```python
from build123d import *

# Parameters (mm, degrees)
SKETCH_1_R          = 9.5
EXTRUDE_1_DEPTH     = 8
SKETCH_1_2_R        = 9.5
EXTRUDE_2_DEPTH     = 8
SKETCH_2_R          = 12
CUT_EXTRUDE_1_DEPTH = 6
SKETCH_3_W          = 20.5
SKETCH_3_H          = 27
CUT_EXTRUDE_2_DEPTH = 4
SKETCH_4_R          = 1.25
CUT_EXTRUDE_3_DEPTH = 5
SKETCH_5_R          = 1.25
CUT_EXTRUDE_4_DEPTH = 7
SKETCH_6_R          = 1.25
CUT_EXTRUDE_5_DEPTH = 7


with BuildPart() as part:
    # Sketch 1 → Extrude 1 (new body)
    with BuildSketch(Plane(origin=(0, 0, 0), x_dir=(1, 0, 0), z_dir=(0, 1, 0))):
        Polygon((-20.5, -13.5), (-20.5, -7.5), (-16.5, -3.5), (-16.5, 3.5), (-20.5, 7.5), (-20.5, 13.5), (41, 13.5), (41, -13.5), align=None)
        with Locations(Location((0, 0, 0), (0, 0, 270))):  # turned: the seam where the file's is
            Circle(SKETCH_1_R, mode=Mode.SUBTRACT)
    extrude(amount=EXTRUDE_1_DEPTH)

    # Sketch 1_2 → Extrude 2 (add)
    with BuildSketch(Plane(origin=(0, 0, 0), x_dir=(1, 0, 0), z_dir=(0, 1, 0))):
        Polygon((-20.5, -13.5), (-20.5, -7.5), (-16.5, -3.5), (-16.5, 3.5), (-20.5, 7.5), (-20.5, 13.5), (41, 13.5), (41, -13.5), align=None)
        with Locations(Location((0, 0, 0), (0, 0, 270))):  # turned: the seam where the file's is
            Circle(SKETCH_1_2_R, mode=Mode.SUBTRACT)
    extrude(amount=EXTRUDE_2_DEPTH)

    # Sketch 2 → Cut-Extrude 1 (cut)
    with BuildSketch(Plane(origin=(0, 8, 0), x_dir=(1, 0, 0), z_dir=(0, 1, 0))):
        with Locations(Location((0, 0, 0), (0, 0, 270))):  # turned: the seam where the file's is
            Circle(SKETCH_2_R)
    extrude(amount=-CUT_EXTRUDE_1_DEPTH, mode=Mode.SUBTRACT)

    # Sketch 3 → Cut-Extrude 2 (cut)
    with BuildSketch(Plane.XZ):
        with Locations((30.75, 0)):
            Rectangle(SKETCH_3_W, SKETCH_3_H)
    extrude(amount=-CUT_EXTRUDE_2_DEPTH, mode=Mode.SUBTRACT)

    # Sketch 4 → Cut-Extrude 3 (cut, through all)
    with BuildSketch(Plane.XZ.offset(-4)):
        with Locations(Location((37, 7.5, 0), (0, 0, 270))):  # turned: the seam where the file's is
            Circle(SKETCH_4_R)
        with Locations(Location((37, -7.5, 0), (0, 0, 90))):  # turned: the seam where the file's is
            Circle(SKETCH_4_R)
    extrude(amount=-CUT_EXTRUDE_3_DEPTH, mode=Mode.SUBTRACT)

    # Sketch 5 → Cut-Extrude 4 (cut)
    with BuildSketch(Plane.XY.offset(13.5)):
        with Locations((-16.5, 3.500018951)):
            Circle(SKETCH_5_R)
        with Locations(Location((16.5, 3.500018951, 0), (0, 0, 180))):  # turned: the seam where the file's is
            Circle(SKETCH_5_R)
    extrude(amount=-CUT_EXTRUDE_4_DEPTH, mode=Mode.SUBTRACT)

    # Sketch 6 → Cut-Extrude 5 (cut)
    with BuildSketch(Plane(origin=(0, 0, -13.5), x_dir=(-1, 0, 0), z_dir=(0, 0, -1))):
        with Locations((16.5, 4)):
            Circle(SKETCH_6_R)
        with Locations(Location((-16.5, 4, 0), (0, 0, 180))):  # turned: the seam where the file's is
            Circle(SKETCH_6_R)
    extrude(amount=-CUT_EXTRUDE_5_DEPTH, mode=Mode.SUBTRACT)


solid = part.part
```
The listing builds one solid part. Answer for the finished solid, in the listing's coordinates (mm). A direction names the side the tool comes from. Give positions to 0.01 mm unless a question says otherwise; leave off trailing zeros. Order: outer loops, then holes, each group sorted by start corner. A loop starts at its lowest first (then second) coordinate and runs counter-clockwise, first axis right, second up. Notation, with made-up numbers: (75.5, 88) - (86.5, 88) arc R18 ccw to (86.5, 97) - close; hole circle Ø11 at (-6, 56). An arc over 180 degrees is marked (long way). Answer in a Markdown table with one row per item. Add a question column.
Q1. Given P1, Ø10, axis at x = 5.5, z = 3.5, coming from the +Y side; P2, Ø1.2, axis at y = 2.5, z = 3.5, coming from the +X side; P3, Ø3, axis at x = -16.5, y = 3.5, coming from the -Z side; P4, Ø3, axis at x = 37, z = 7.5, coming from the -Y side, each flat-ended and moving along its own axis, determine where each tip first touches the part or whether it passes through.
Q2. Find the intervals of material crossed by line 1 along X through (y, z) = (0.7, 0); line 2 along X through (y, z) = (5.3, -7.5); line 3 along X through (y, z) = (6.4, 0), in increasing order. Write a range as [from, to].
Q3. The part is cut by section C-C (z = 0). Determine the outline of the cut face in (x, y), then the cut area to 3 significant figures.
Q4. For a pull along Y with two mould halves and no side action, classify faces 5 (the flat face through (17, 3, 6.5)), 6 (the flat face through (-20.5, 4, -10)), 7 (the flat face through (18, 8, 0)) as released by +Y, released by -Y, zero draft, split by the parting line, or undercut.
Q5. Which of the six approach directions +Z, -Z, +X, -X, +Y, -Y give full straight-line access (tool end or side, diameter ignored) to faces 1 (the cylindrical face through (16.23, 5.22, -10.05)), 2 (the flat face through (31, 4, 0)), 3 (the flat face through (-19, 4, 6)), 4 (the cylindrical face through (-16.77, 2.28, 10.05))?
Q6. The part is cut by section B-B (y = 7.25). Determine the outline of the cut face in (x, z).
Q7. The part is cut by section A-A (x = 37). Determine the outline of the cut face in (y, z).
Q8. The part is cut by section D-D (x = 16.5). Determine the outline of the cut face in (y, z), then the cut area to 3 significant figures.
Determined:
| question | item | result |
|---|---|---|
| 1 | P1 | stops at y = 2 |
| 1 | P2 | stops at x = 20.5 |
| 1 | P3 | stops at z = -13.5 |
| 1 | P4 | stops at y = 4 |
| 2 | line 1 | x = [-16.5, -9.5], [9.5, 20.5] |
| 2 | line 2 | x = [-20.5, -9.37], [9.37, 35.75], [38.25, 41] |
| 2 | line 3 | x = [-16.5, -12], [12, 41] |
| 3 | outline | (-16.5, 0) - (-9.5, 0) - (-9.5, 2) - (-12, 2) - (-12, 8) - (-16.5, 8) - close; (9.5, 0) - (20.5, 0) - (20.5, 4) - (41, 4) - (41, 8) - (12, 8) - (12, 2) - (9.5, 2) - close |
| 3 | area | 196 mm² |
| 4 | face 5 | undercut |
| 4 | face 6 | zero draft |
| 4 | face 7 | released by +Y |
| 5 | face 1 | -Z |
| 5 | face 2 | +Z, -Z, +X, -Y |
| 5 | face 3 | -X, +Y, -Y |
| 5 | face 4 | +Z |
| 6 | outline | (-20.5, -13.5) - (41, -13.5) - (41, 13.5) - (-20.5, 13.5) - (-20.5, 7.5) - (-16.5, 3.5) - (-16.5, -3.5) - (-20.5, -7.5) - close; hole circle Ø24 at (0, 0); hole circle Ø2.5 at (37, -7.5); hole circle Ø2.5 at (37, 7.5) |
| 7 | outline | (4, -13.5) - (8, -13.5) - (8, -8.75) - (4, -8.75) - close; (4, -6.25) - (8, -6.25) - (8, 6.25) - (4, 6.25) - close; (4, 8.75) - (8, 8.75) - (8, 13.5) - (4, 13.5) - close |
| 8 | outline | (0, -13.5) - (2.75, -13.5) - (2.75, -6.5) - (5.25, -6.5) - (5.25, -13.5) - (8, -13.5) - (8, 13.5) - (4.75, 13.5) - (4.75, 6.5) - (2.25, 6.5) - (2.25, 13.5) - (0, 13.5) - close |
| 8 | area | 181 mm² |
